For this review, take the finished solid that the model builds, in its own axes (mm). Give positions to 0.01 mm unless a question says otherwise; leave off trailing zeros. Loops run counter-clockwise (first coordinate to the right, second up) from the corner with the lowest first, then second, coordinate; pieces in that order, holes last. Notation, with made-up numbers: (62.5, 8) - (93.5, 8) arc R24 ccw to (93.5, 27) - close; hole circle Ø3 at (-26, 24.25). An arc over 180 degrees is marked (long way). Answer in a Markdown table with one row per item.
```python
from build123d import *

# Parameters (mm, degrees)
SKETCH_1_R               = 32.5
SKETCH_1_R_2             = 2.55
SKETCH_1_R_3             = 13.1
EXTRUDE_1_DEPTH          = 3
HOLE_WIZARD_1_AT_2_COUNT = 2
HOLE_WIZARD_1_AT_2_PITCH = 43.301270189
HOLE_WIZARD_1_AT_3_COUNT = 2
HOLE_WIZARD_1_AT_3_PITCH = 43.301270189


with BuildPart() as part:
    # 草图1 → 凸台-拉伸1 (new body)
    with BuildSketch(Plane.XY):
        Circle(SKETCH_1_R)
        with Locations((0, 17.5)):
            Circle(SKETCH_1_R_2, mode=Mode.SUBTRACT)
        with Locations((15.155444566, -8.75)):
            Circle(SKETCH_1_R_2, mode=Mode.SUBTRACT)
        with Locations((-15.155444566, -8.75)):
            Circle(SKETCH_1_R_2, mode=Mode.SUBTRACT)
        with Locations((21.650635095, 12.5)):
            Circle(SKETCH_1_R_2, mode=Mode.SUBTRACT)
        with Locations((0, -25)):
            Circle(SKETCH_1_R_2, mode=Mode.SUBTRACT)
        with Locations((-21.650635095, 12.5)):
            Circle(SKETCH_1_R_2, mode=Mode.SUBTRACT)
        Circle(SKETCH_1_R_3, mode=Mode.SUBTRACT)
    extrude(amount=EXTRUDE_1_DEPTH)

    # 草图3 → 打孔尺寸(%根据十字)槽沉头木螺钉的类型1 (revolve, cut)
    with BuildSketch(Plane(origin=(21.650635095, 12.5, 0), x_dir=(0, 1, 0), z_dir=(1, 0, 0))):
        Polygon((0, 0), (0, 3), (2.5, 3), (2.5, 3.1), (5.6, 0), align=None)
    hole_wizard_1 = revolve(axis=Axis((21.650635095, 12.5, -6.35), (0, 0, 1)), mode=Mode.SUBTRACT)

    # 打孔尺寸(%根据十字)槽沉头木螺钉的类型1 at 2: 打孔尺寸(%根据十字)槽沉头木螺钉的类型1 ×2
    with Locations(*[(-i * HOLE_WIZARD_1_AT_2_PITCH, 0, 0) for i in range(1, HOLE_WIZARD_1_AT_2_COUNT)]):
        add(hole_wizard_1, mode=Mode.SUBTRACT)

    # 打孔尺寸(%根据十字)槽沉头木螺钉的类型1 at 3: 打孔尺寸(%根据十字)槽沉头木螺钉的类型1 ×2
    with Locations(*[Vector(-0.5000000000000018, -0.8660254037844376, 0) * (i * HOLE_WIZARD_1_AT_3_PITCH) for i in range(1, HOLE_WIZARD_1_AT_3_COUNT)]):
        add(hole_wizard_1, mode=Mode.SUBTRACT)


solid = part.part
```
1. Clearance check with flat-ended pins moving along their axes: pin 1 (3 mm diameter, centred on x = -15.16, y = -8.75, fed in from +Z); pin 2 (1.5 mm diameter, centred on x = 0, z = 0.5, fed in from -Y). State where each tip first meets the part, or that it passes through.
Values:
| item | result |
|---|---|
| pin 1 | passes through |
| pin 2 | stops at y = -32.5 |
2. Wall thickness on line 1 (X direction, y = 14, z = 1.3); line 2 (X direction, y = 11, z = 0.55); line 3 (X direction, y = 14, z = 2.7): over which ranges is each line inside the solid? List them lowest first. Write a range as [from, to].
Values:
| item | result |
|---|---|
| line 1 | x = [-29.33, -25.68], [-17.62, 17.62], [25.68, 29.33] |
| line 2 | x = [-30.58, -26.47], [-16.83, -7.11], [7.11, 16.83], [26.47, 30.58] |
| line 3 | x = [-29.33, -24.13], [-19.17, 19.17], [24.13, 29.33] |
3. We need section D-D, the plane x = 1. Count the separate pieces of the cut face and the enclosed holes in it, and give its area (3 significant figures).
Values:
| item | result |
|---|---|
| separate pieces | 4 |
| enclosed holes | 0 |
| area | 78.6 mm^2 |
4. We need section B-B, the plane z = 2.2. Give the boundary of the cut face in (x, y).
Values:
| item | result |
|---|---|
| outline | circle Ø65 at (0, 0); hole circle Ø6.8 at (-21.65, 12.5); hole circle Ø5.1 at (-15.16, -8.75); hole circle Ø26.2 at (0, 0); hole circle Ø6.8 at (0, -25); hole circle Ø5.1 at (0, 17.5); hole circle Ø5.1 at (15.16, -8.75); hole circle Ø6.8 at (21.65, 12.5) |
5. We need section C-C, the plane y = -25. Give the boundary of the cut face in (x, z).
Values:
| item | result |
|---|---|
| outline | (-20.77, 0) - (-5.6, 0) - (-2.6, 3) - (-20.77, 3) - close; (2.6, 3) - (5.6, 0) - (20.77, 0) - (20.77, 3) - close |
6. We need section A-A, the plane y = 0. Give the boundary of the cut face in (x, z), and give its area (3 significant figures).
Values:
| item | result |
|---|---|
| outline | (-32.5, 0) - (-13.1, 0) - (-13.1, 3) - (-32.5, 3) - close; (13.1, 0) - (32.5, 0) - (32.5, 3) - (13.1, 3) - close |
| area | 116 mm^2 |
7. Mouldability with a two-part tool opening along Y and no side actions: class faces 1 (the face through (14, 0, 0)), 2 (the face through (31, 9.76, 1.48)), 3 (the face through (1.18, 15.24, 1.48)) as released by +Y, released by -Y, zero draft, split by the parting line, or undercut.
Values:
| item | result |
|---|---|
| face 1 | zero draft |
| face 2 | split by the parting line |
| face 3 | undercut |
